Verification items for the finished model (mm, model axes). A direction names the side the tool comes from. Coordinates: 2 decimals unless noted, no trailing zeros. Order: outer loops, then holes, each group sorted by start corner. A loop starts at its lowest first (then second) coordinate and runs counter-clockwise, first axis right, second up. Notation, with made-up numbers: M -15.75,59 L 17.25,59 A29 ccw 17.25,98 Z; hole C 42.5,24 d2. An arc over 180 degrees is marked long. Return JSON: item names as keys, results as strings.
```python
from build123d import *

# Parameters (mm, degrees)
SKETCH1_W                   = 6.35
SKETCH1_H                   = 57.15
SKETCH1_W_2                 = 88.9
SKETCH1_H_2                 = 6.35
BOSS_EXTRUDE1_DEPTH         = 92.86494
MASTER_CYLINDER_MOUNT_REACH = 59.15
SKETCH2_R                   = 5.08
SKETCH2_R_2                 = 20.32
SKETCH3_R                   = 3.96875
BRACKET_MOUNT_DEPTH         = 102.6


with BuildPart() as part:
    # Sketch1 → Boss-Extrude1 (new body)
    with BuildSketch(Plane.XY):
        with Locations((-109.443697604, 28.678448761)):
            Rectangle(SKETCH1_W, SKETCH1_H)
        with Locations((-61.818697604, 54.078448761)):
            Rectangle(SKETCH1_W_2, SKETCH1_H_2)
        Polygon((-17.368697604, 57.253448761), (-17.368697604, 50.903448761), (-17.368697604, 0.103448761), (-11.018697604, 0.103448761), (-11.018697604, 57.253448761), align=None)
    extrude(amount=BOSS_EXTRUDE1_DEPTH)

    # Sketch2 → Master Cylinder Mount (cut, up to next)
    with BuildSketch(Plane(origin=(0, 57.253448761, 0), x_dir=(1, 0, 0), z_dir=(0, 1, 0)), mode=Mode.PRIVATE) as master_cylinder_mount_sk1:
        Polygon((-47.531197604, 0), (-76.106197604, 0), (-76.106197604, -13.97), (-69.121197604, -13.97), (-54.516197604, -13.97), (-47.531197604, -13.97), align=None)
    master_cylinder_mount_tool1 = extrude(master_cylinder_mount_sk1.sketch, amount=-MASTER_CYLINDER_MOUNT_REACH, mode=Mode.PRIVATE) & part.part
    add(master_cylinder_mount_tool1.solids().sort_by_distance((-61.818698, 57.253449, 6.985))[0], mode=Mode.SUBTRACT)
    # Sketch2 → Master Cylinder Mount (cut, up to next)
    with BuildSketch(Plane(origin=(0, 57.253448761, 0), x_dir=(1, 0, 0), z_dir=(0, 1, 0)), mode=Mode.PRIVATE) as master_cylinder_mount_sk2:
        with Locations((-38.958697604, -26.18994)):
            Circle(SKETCH2_R)
    master_cylinder_mount_tool2 = extrude(master_cylinder_mount_sk2.sketch, amount=-MASTER_CYLINDER_MOUNT_REACH, mode=Mode.PRIVATE) & part.part
    add(master_cylinder_mount_tool2.solids().sort_by_distance((-38.958698, 57.253449, 26.18994))[0], mode=Mode.SUBTRACT)
    # Sketch2 → Master Cylinder Mount (cut, up to next)
    with BuildSketch(Plane(origin=(0, 57.253448761, 0), x_dir=(1, 0, 0), z_dir=(0, 1, 0)), mode=Mode.PRIVATE) as master_cylinder_mount_sk3:
        with Locations((-84.678697604, -26.18994)):
            Circle(SKETCH2_R)
    master_cylinder_mount_tool3 = extrude(master_cylinder_mount_sk3.sketch, amount=-MASTER_CYLINDER_MOUNT_REACH, mode=Mode.PRIVATE) & part.part
    add(master_cylinder_mount_tool3.solids().sort_by_distance((-84.678698, 57.253449, 26.18994))[0], mode=Mode.SUBTRACT)
    # Sketch2 → Master Cylinder Mount (cut, up to next)
    with BuildSketch(Plane(origin=(0, 57.253448761, 0), x_dir=(1, 0, 0), z_dir=(0, 1, 0)), mode=Mode.PRIVATE) as master_cylinder_mount_sk4:
        with Locations((-84.678697604, -83.33994)):
            Circle(SKETCH2_R)
    master_cylinder_mount_tool4 = extrude(master_cylinder_mount_sk4.sketch, amount=-MASTER_CYLINDER_MOUNT_REACH, mode=Mode.PRIVATE) & part.part
    add(master_cylinder_mount_tool4.solids().sort_by_distance((-84.678698, 57.253449, 83.33994))[0], mode=Mode.SUBTRACT)
    # Sketch2 → Master Cylinder Mount (cut, up to next)
    with BuildSketch(Plane(origin=(0, 57.253448761, 0), x_dir=(1, 0, 0), z_dir=(0, 1, 0)), mode=Mode.PRIVATE) as master_cylinder_mount_sk5:
        with Locations((-38.958697604, -83.33994)):
            Circle(SKETCH2_R)
    master_cylinder_mount_tool5 = extrude(master_cylinder_mount_sk5.sketch, amount=-MASTER_CYLINDER_MOUNT_REACH, mode=Mode.PRIVATE) & part.part
    add(master_cylinder_mount_tool5.solids().sort_by_distance((-38.958698, 57.253449, 83.33994))[0], mode=Mode.SUBTRACT)
    # Sketch2 → Master Cylinder Mount (cut, up to next)
    with BuildSketch(Plane(origin=(0, 57.253448761, 0), x_dir=(1, 0, 0), z_dir=(0, 1, 0)), mode=Mode.PRIVATE) as master_cylinder_mount_sk6:
        with Locations((-38.958697604, -54.76494)):
            Circle(SKETCH2_R_2)
    master_cylinder_mount_tool6 = extrude(master_cylinder_mount_sk6.sketch, amount=-MASTER_CYLINDER_MOUNT_REACH, mode=Mode.PRIVATE) & part.part
    add(master_cylinder_mount_tool6.solids().sort_by_distance((-38.958698, 57.253449, 54.76494))[0], mode=Mode.SUBTRACT)
    # Sketch2 → Master Cylinder Mount (cut, up to next)
    with BuildSketch(Plane(origin=(0, 57.253448761, 0), x_dir=(1, 0, 0), z_dir=(0, 1, 0)), mode=Mode.PRIVATE) as master_cylinder_mount_sk7:
        with Locations((-84.678697604, -54.76494)):
            Circle(SKETCH2_R_2)
    master_cylinder_mount_tool7 = extrude(master_cylinder_mount_sk7.sketch, amount=-MASTER_CYLINDER_MOUNT_REACH, mode=Mode.PRIVATE) & part.part
    add(master_cylinder_mount_tool7.solids().sort_by_distance((-84.678698, 57.253449, 54.76494))[0], mode=Mode.SUBTRACT)

    # Sketch3 → Bracket Mount (cut, through all)
    with BuildSketch(Plane.ZY.offset(112.618697604)):
        with Locations((19.05, 12.803448761)):
            Circle(SKETCH3_R)
        with Locations((19.05, 31.853448761)):
            Circle(SKETCH3_R)
    extrude(amount=-BRACKET_MOUNT_DEPTH, mode=Mode.SUBTRACT)


solid = part.part
```
Q1. Cross-section at A-A, the plane z = 19.05. Record the boundary of the cut face in (x, y).
Values:
{"outline": "M -112.62,0.1 L -106.27,0.1 L -106.27,8.83 L -112.62,8.83 Z; M -112.62,16.77 L -106.27,16.77 L -106.27,27.88 L -112.62,27.88 Z; M -112.62,35.82 L -106.27,35.82 L -106.27,50.9 L -17.37,50.9 L -17.37,35.82 L -11.02,35.82 L -11.02,57.25 L -112.62,57.25 Z; M -17.37,0.1 L -11.02,0.1 L -11.02,8.83 L -17.37,8.83 Z; M -17.37,16.77 L -11.02,16.77 L -11.02,27.88 L -17.37,27.88 Z"}
Q2. Material ranges on line 1 along Y through (x, z) = (-110.5, 19.05); line 2 along X through (y, z) = (50.5, 44); line 3 along Y through (x, z) = (-49, 36), recorded low to high.
Values:
{"line 1": "0.1 to 8.83, 16.77 to 27.88, 35.82 to 57.25", "line 2": "-112.62 to -106.27, -17.37 to -11.02", "line 3": "50.9 to 57.25"}
Q3. Cross-section at C-C, the plane z = 64. Record the boundary of the cut face in (x, y).
Values:
{"outline": "M -112.62,0.1 L -106.27,0.1 L -106.27,50.9 L -102.78,50.9 L -102.78,57.25 L -112.62,57.25 Z; M -66.58,50.9 L -57.06,50.9 L -57.06,57.25 L -66.58,57.25 Z; M -20.86,50.9 L -17.37,50.9 L -17.37,0.1 L -11.02,0.1 L -11.02,57.25 L -20.86,57.25 Z"}
Q4. Cross-section at B-B, the plane y = 6.5. Record the boundary of the cut face in (x, z), and give its area (3 significant figures).
Values:
{"outline": "M -112.62,0 L -106.27,0 L -106.27,92.86 L -112.62,92.86 Z; M -17.37,0 L -11.02,0 L -11.02,92.86 L -17.37,92.86 Z", "area": "1,180 mm^2"}
Q5. Cross-section at D-D, the plane x = -68.5. Record the boundary of the cut face in (y, z).
Values:
{"outline": "M 50.9,13.97 L 57.25,13.97 L 57.25,42.47 L 50.9,42.47 Z; M 50.9,67.06 L 57.25,67.06 L 57.25,92.86 L 50.9,92.86 Z"}
Q6. Tool access check on faces 1 (the face through (-17.369, 26, 46)), 2 (the face through (-107, 37, 0)), 3 (the face through (-76.106, 54, 7)). Record the directions out of +Z, -Z, +X, -X, +Y, -Y that give a thin tool (end or side, any length) a straight path to the whole face; none if there is none.
Values:
{"face 1": "+Z, -Z, -Y", "face 2": "-Z, +X, -X, +Y, -Y", "face 3": "-Z, +Y, -Y"}
Q7. Draft check along Y on faces 4 (the face through (-61, 57.253, 46)), 5 (the face through (-14, 0.103, 46)), 6 (the face through (-14.24, 29.44, 15.9)), 7 (the face through (-79.833, 54.123, 24.664)). Enter one of: pulls with the +Y half, pulls with the -Y half, needs draft (parallel to the pull), parting line crosses it, or undercut.
Values:
{"face 4": "pulls with the +Y half", "face 5": "pulls with the -Y half", "face 6": "undercut", "face 7": "needs draft"}
Q8. Go/stop test with flat-tipped pins: pin 1 (16.5 mm diameter, centred on x = -84.68, z = 26.19, fed in from -Y); pin 2 (6.5 mm diameter, centred on y = 12.8, z = 19.05, fed in from +X); pin 3 (5 mm diameter, centred on x = -57, y = 52.5, fed in from -Z). Record where each tip stops, or that it passes through.
Values:
{"pin 1": "y = 50.9", "pin 2": "through", "pin 3": "z = 13.97"}
